```python
from build123d import *

# Parameters (mm, degrees)
SKETCH1_W           = 28
SKETCH1_H           = 22
BOSS_EXTRUDE1_DEPTH = 1.69
SKETCH2_R           = 1.445350302
SKETCH2_R_2         = 1.385905996
SKETCH2_R_3         = 1.453223353
SKETCH2_R_4         = 1.406338145
CUT_EXTRUDE1_DEPTH  = 1.69
SKETCH3_W           = 5
SKETCH3_H           = 5
BOSS_EXTRUDE2_DEPTH = 1
SKETCH4_W           = 2.5
SKETCH4_H           = 8
BOSS_EXTRUDE3_DEPTH = 2
SKETCH5_W           = 3
SKETCH5_H           = 5
CUT_EXTRUDE2_DEPTH  = 10


with BuildPart() as part:
    # Sketch1 → Boss-Extrude1 (new body)
    with BuildSketch(Plane.XY):
        with Locations((14, 11)):
            Rectangle(SKETCH1_W, SKETCH1_H)
    extrude(amount=BOSS_EXTRUDE1_DEPTH)

    # Sketch2 → Cut-Extrude1 (cut)
    with BuildSketch(Plane.XY.offset(1.69)):
        with Locations((26, 19.834515058)):
            Circle(SKETCH2_R)
        with Locations((26, 1.826288901)):
            Circle(SKETCH2_R_2)
        with Locations((15, 1.826288901)):
            Circle(SKETCH2_R_3)
        with Locations((15, 19.834515058)):
            Circle(SKETCH2_R_4)
    extrude(amount=-CUT_EXTRUDE1_DEPTH, mode=Mode.SUBTRACT)

    # Sketch3 → Boss-Extrude2 (add)
    with BuildSketch(Plane.XY.offset(1.69)):
        with Locations((20.5, 10.83040198)):
            Rectangle(SKETCH3_W, SKETCH3_H)
    extrude(amount=BOSS_EXTRUDE2_DEPTH)

    # Sketch4 → Boss-Extrude3 (add)
    with BuildSketch(Plane.XY.offset(1.69)):
        with Locations((10.5, 12)):
            Rectangle(SKETCH4_W, SKETCH4_H)
    extrude(amount=BOSS_EXTRUDE3_DEPTH)

    # Sketch5 → Cut-Extrude2 (cut)
    with BuildSketch(Plane.XY.offset(1.69)):
        with Locations((1.5, 2.5)):
            Rectangle(SKETCH5_W, SKETCH5_H)
    extrude(amount=-CUT_EXTRUDE2_DEPTH, mode=Mode.SUBTRACT)


solid = part.part
```
Model file for the job. Use its own axes, mm. A direction names the side the tool comes from. Give positions to 0.01 mm unless a question says otherwise; leave off trailing zeros. Loops run counter-clockwise (first coordinate to the right, second up) from the corner with the lowest first, then second, coordinate; pieces in that order, holes last. Notation, with made-up numbers: (28.5, 87.5) -> (42.5, 87.5) arc R12 cw to (42.5, 91.5) -> close; hole circle Ø9 at (11, 54.25). An arc over 180 degrees is marked (long way). Use CSV: the item, a comma, the result in double quotes. Start each with the question number.
1) Tool access for faces 4 (the flat face through (10, 8, 3)), 5 (the flat face through (9.25, 12, 3)), 6 (the flat face through (10, 16, 3)), 7 (the flat face through (11.75, 12, 3)), 8 (the flat face through (20, 13.33, 2)): list every direction of +Z, -Z, +X, -X, +Y, -Y with a clear straight run to the whole face (end or side of a thin tool).
2) Slice it at B-B on y = 12.25. Give the cut face in (x, z).
3) Slice it at C-C on z = 0.3. Give the cut face in (x, y), plus the area to 3 significant figures.
4) Slice it at D-D on x = 26. Give the cut face in (y, z), plus the area to 3 significant figures.
5) Flat gauge pins, fed straight in: pin 1 Ø1.5 at (x, y) = (19.5, 10) entering from +Z; pin 2 Ø1.6 at (x, z) = (11, 3) entering from -Y; pin 3 Ø4 at (x, y) = (14.5, 6) entering from +Z. Where does each tip first touch, or does it go through?
6) Wall check: line 1 (Y direction, x = 26, z = 0.9); line 2 (Y direction, x = 15, z = 0.4); line 3 (X direction, y = 12.75, z = 1.9). Give the ranges that are in metal, low to high.
7) Mould opens along X. For faces 1 (the flat face through (0, 13, 1)), 2 (the flat face through (18, 11, 2)), 3 (the flat face through (14, 11, 0)) say: released by +X, released by -X, zero draft, split by the parting line, or undercut.
8) Slice it at A-A on x = 15. Give the cut face in (y, z), plus the area to 3 significant figures.
Computed values:
1,face 4,"+Z, +X, -X, -Y"
1,face 5,"+Z, -X, +Y, -Y"
1,face 6,"+Z, +X, -X, +Y"
1,face 7,"+Z, +Y, -Y"
1,face 8,"+Z, +X, +Y"
2,outline,"(0, 0) -> (28, 0) -> (28, 1.69) -> (23, 1.69) -> (23, 2.69) -> (18, 2.69) -> (18, 1.69) -> (11.75, 1.69) -> (11.75, 3.69) -> (9.25, 3.69) -> (9.25, 1.69) -> (0, 1.69) -> close"
3,outline,"(0, 5) -> (3, 5) -> (3, 0) -> (28, 0) -> (28, 22) -> (0, 22) -> close; hole circle Ø2.91 at (15, 1.83); hole circle Ø2.81 at (15, 19.83); hole circle Ø2.89 at (26, 19.83); hole circle Ø2.77 at (26, 1.83)"
3,area,"576 mm^2"
4,outline,"(0, 0) -> (0.44, 0) -> (0.44, 1.69) -> (0, 1.69) -> close; (3.21, 0) -> (18.39, 0) -> (18.39, 1.69) -> (3.21, 1.69) -> close; (21.28, 0) -> (22, 0) -> (22, 1.69) -> (21.28, 1.69) -> close"
4,area,"27.6 mm^2"
5,pin 1,"stops at z = 2.69"
5,pin 2,"stops at y = 8"
5,pin 3,"stops at z = 1.69"
6,line 1,"y = 0 to 0.44, 3.21 to 18.39, 21.28 to 22"
6,line 2,"y = 0 to 0.37, 3.28 to 18.43, 21.24 to 22"
6,line 3,"x = 9.25 to 11.75, 18 to 23"
7,face 1,"released by -X"
7,face 2,"undercut"
7,face 3,"zero draft"
8,outline,"(0, 0) -> (0.37, 0) -> (0.37, 1.69) -> (0, 1.69) -> close; (3.28, 0) -> (18.43, 0) -> (18.43, 1.69) -> (3.28, 1.69) -> close; (21.24, 0) -> (22, 0) -> (22, 1.69) -> (21.24, 1.69) -> close"
8,area,"27.5 mm^2"
